```python
from build123d import *

# Parameters (mm, degrees)
SKETCH013_W     = 40
SKETCH013_H     = 40
PAD002_DEPTH    = 13
SKETCH014_W     = 20
SKETCH014_H     = 19.786463
POCKET008_DEPTH = 30
SKETCH015_R     = 11
POCKET009_DEPTH = 13.001
SKETCH017_R     = 1.75
POCKET010_DEPTH = 13.001
SKETCH018_R     = 1.9
POCKET011_DEPTH = 5
SKETCH019_R     = 2.75
POCKET012_DEPTH = 5
CHAMFER002_SIZE = 0.9
CHAMFER005_SIZE = 2


with BuildPart() as part:
    # Sketch013 → Pad002 (new body)
    with BuildSketch(Plane.XY):
        Rectangle(SKETCH013_W, SKETCH013_H)
    extrude(amount=PAD002_DEPTH)

    # Sketch014 (on Face4 of Pad002) → Pocket008 (cut)
    with BuildSketch(Plane(origin=(-20, 0, 0), x_dir=(0, -1, 0), z_dir=(-1, 0, 0))):
        with Locations((0, -1.893231)):
            Rectangle(SKETCH014_W, SKETCH014_H)
    extrude(amount=-POCKET008_DEPTH, mode=Mode.SUBTRACT)

    # Sketch015 (on Face5 of Pocket008) → Pocket009 (cut, through all)
    with BuildSketch(Plane.XY.offset(13)):
        Circle(SKETCH015_R)
    extrude(amount=-POCKET009_DEPTH, mode=Mode.SUBTRACT)

    # Sketch017 (on Face5 of Pocket009) → Pocket010 (cut, through all)
    with BuildSketch(Plane.XY.offset(13)):
        with Locations((0, 15.5)):
            Circle(SKETCH017_R)
        with Locations((15.5, 0)):
            Circle(SKETCH017_R)
        with Locations((0, -15.5)):
            Circle(SKETCH017_R)
        with Locations((-15.5, 15.5)):
            Circle(SKETCH017_R)
        with Locations((15.5, 15.5)):
            Circle(SKETCH017_R)
        with Locations((-15.5, -15.5)):
            Circle(SKETCH017_R)
        with Locations((15.5, -15.5)):
            Circle(SKETCH017_R)
    extrude(amount=-POCKET010_DEPTH, mode=Mode.SUBTRACT)

    # Sketch018 → Pocket011 (cut)
    with BuildSketch(Plane.XY.offset(20)):
        with Locations((0, 15.5)):
            Circle(SKETCH018_R)
        with Locations((15.5, 0)):
            Circle(SKETCH018_R)
        with Locations((0, -15.5)):
            Circle(SKETCH018_R)
    extrude(amount=-POCKET011_DEPTH, mode=Mode.SUBTRACT)

    # Sketch019 → Pocket012 (cut)
    with BuildSketch(Plane(origin=(0, 0, 0), x_dir=(1, 0, 0), z_dir=(0, 0, -1))):
        with Locations((-15.5, 15.5)):
            Circle(SKETCH019_R)
        with Locations((15.5, 15.5)):
            Circle(SKETCH019_R)
        with Locations((15.5, -15.5)):
            Circle(SKETCH019_R)
        with Locations((-15.5, -15.5)):
            Circle(SKETCH019_R)
    extrude(amount=-POCKET012_DEPTH, mode=Mode.SUBTRACT)

    # Chamfer002
    chamfer002_edges = [part.edges().sort_by_distance(p)[0] for p in [
        (1.75, -15.5, 6.5),
        (-18.25, 15.5, 5),
        (18.25, 15.5, 2.5),
    ]]
    chamfer(chamfer002_edges, length=CHAMFER002_SIZE)

    # Chamfer005
    chamfer005_edges = [part.edges().sort_by_distance(p)[0] for p in [
        (-20, 20, 6.5),
        (20, 20, 6.5),
        (20, -20, 6.5),
        (-20, -20, 6.5),
    ]]
    chamfer(chamfer005_edges, length=CHAMFER005_SIZE)


solid = part.part
```
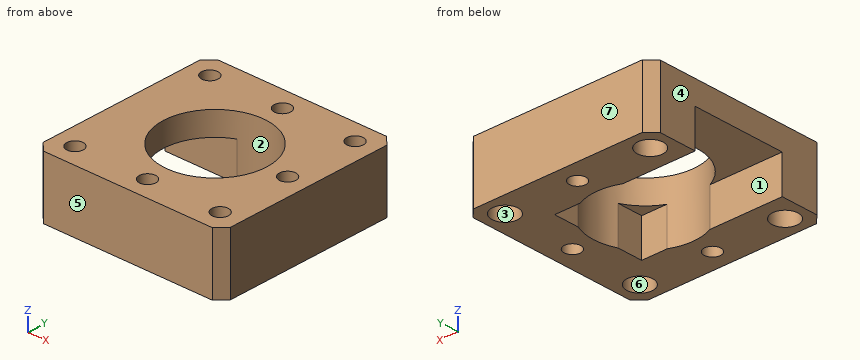
CAD build for the part. Positions are in the model's coordinates, mm. Face numbers are marked on the shaded views. A direction names the side the tool comes from. Round coordinates to 2 decimals unless told otherwise and drop trailing zeros. Order: outer loops, then holes, each group sorted by start corner. A loop starts at its lowest first (then second) coordinate and runs counter-clockwise, first axis right, second up.
Item 1: Mould opens along Y. For the marked faces 4, 5, 6 and 7 say: pulls with the +Y half, pulls with the -Y half, needs draft (parallel to the pull), parting line crosses it, or undercut.
Item 2: Saw through at A-A on y = 0. Write the cut outline in (x, z).
Item 3: Saw through at D-D on y = -15.5. Write the cut outline in (x, z), then the cut area to 4 significant figures.
Item 4: Saw through at B-B on x = 0. Write the cut outline in (y, z), then the cut area to 3 significant figures.
Item 5: Pin check, flat tips, straight feed: pin 1 (1.6 mm diameter, centred on x = -14.5, y = -16.5, fed in from -Z); pin 2 (3 mm diameter, centred on x = 7, y = 6.5, fed in from -Z); pin 3 (2.5 mm diameter, centred on y = 6.5, z = 3.5, fed in from -X). Stop position of each tip, or through.
Item 6: Probe line 1 along Y through (x, z) = (15.5, 3.7); line 2 along Y through (x, z) = (0, 10); line 3 along Y through (x, z) = (-15.5, 9.25). List the from-to ranges inside material, lowest first.
Item 7: Saw through at C-C on z = 6. Write the cut outline in (x, y), then the cut area to 3 significant figures.
Item 8: Tool access for the marked faces 1, 2 and 3: list every direction of +Z, -Z, +X, -X, +Y, -Y with a clear straight run to the whole face (end or side of a thin tool).
Reported:
1. face 4: needs draft
1. face 5: pulls with the -Y half
1. face 6: undercut
1. face 7: pulls with the +Y half
2. outline: (-20, 8) - (-11, 8) - (-11, 13) - (-20, 13) - close; (11, 0) - (13.75, 0) - (13.75, 13) - (11, 13) - close; (17.25, 0) - (20, 0) - (20, 13) - (17.25, 13) - close
3. outline: (-20, 0) - (-18.25, 0) - (-18.25, 5) - (-17.25, 5) - (-17.25, 13) - (-20, 13) - close; (-13.75, 5) - (-12.75, 5) - (-12.75, 0) - (-1.75, 0) - (-1.75, 13) - (-13.75, 13) - close; (1.75, 0) - (12.75, 0) - (12.75, 5) - (13.75, 5) - (13.75, 13) - (1.75, 13) - close; (17.25, 5) - (18.25, 5) - (18.25, 0) - (20, 0) - (20, 13) - (17.25, 13) - close
3. area: 363.5 mm2
4. outline: (-20, 0) - (-17.25, 0) - (-17.25, 13) - (-20, 13) - close; (-13.75, 0) - (-11, 0) - (-11, 13) - (-13.75, 13) - close; (11, 0) - (13.75, 0) - (13.75, 13) - (11, 13) - close; (17.25, 0) - (20, 0) - (20, 13) - (17.25, 13) - close
4. area: 143 mm2
5. pin 1: stops at z = 5
5. pin 2: stops at z = 8
5. pin 3: stops at x = 10
6. line 1: y = -20 to -18.25, -12.75 to -1.75, 1.75 to 12.75, 18.25 to 20
6. line 2: y = -20 to -17.25, -13.75 to -11, 11 to 13.75, 17.25 to 20
6. line 3: y = -20 to -17.25, -13.75 to 13.75, 17.25 to 20
7. outline: (-20, -18) - (-18, -20) - (18, -20) - (20, -18) - (20, 18) - (18, 20) - (-18, 20) - (-20, 18) - (-20, 10) - (-4.58, 10) arc R11 cw to (4.58, 10) - (10, 10) - (10, 4.58) arc R11 cw to (10, -4.58) - (10, -10) - (4.58, -10) arc R11 cw to (-4.58, -10) - (-20, -10) - close; hole circle Ø3.5 at (-15.5, -15.5); hole circle Ø3.5 at (-15.5, 15.5); hole circle Ø3.5 at (0, -15.5); hole circle Ø3.5 at (0, 15.5); hole circle Ø3.5 at (15.5, -15.5); hole circle Ø3.5 at (15.5, 0); hole circle Ø3.5 at (15.5, 15.5)
7. area: 906 mm2
8. face 1: -Z, -X
8. face 2: +Z, -Z
8. face 3: -Z
